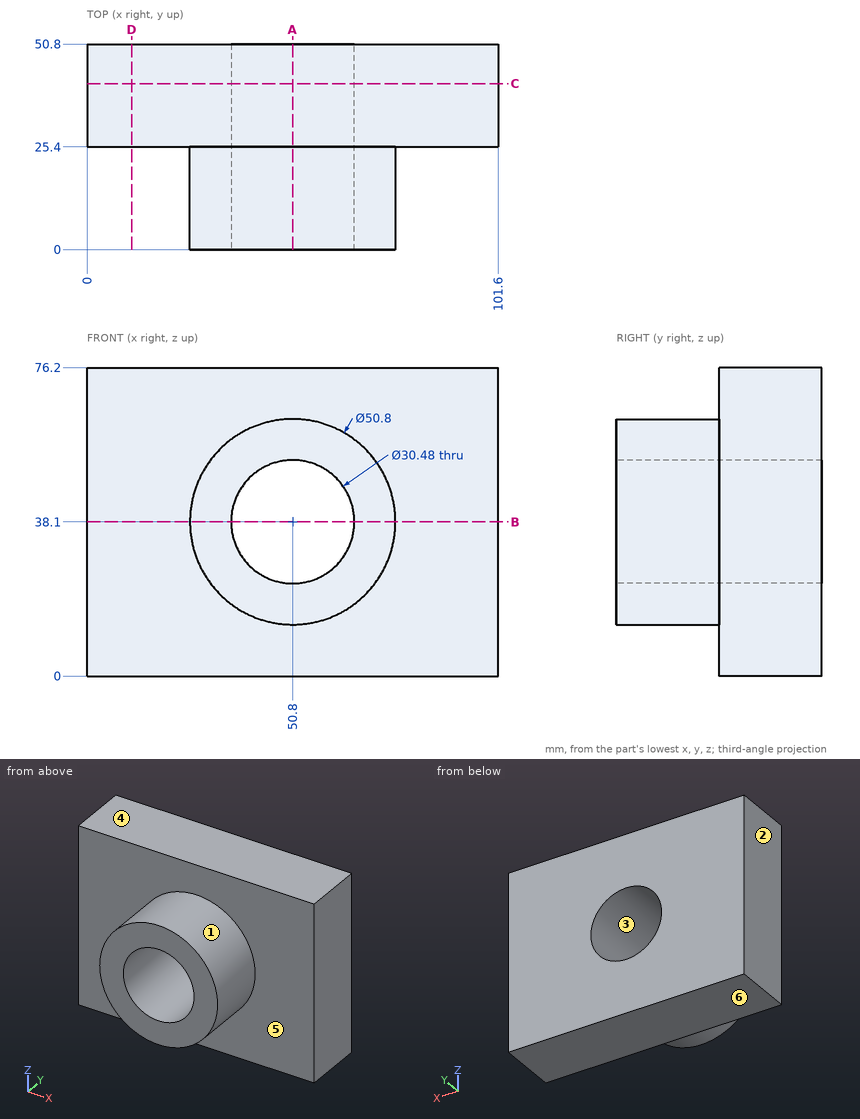
Print and shaded views of the part. All mm, measured from the part's lowest x, y and z. A direction names the side the tool comes from. Round coordinates to 2 decimals unless told otherwise and drop trailing zeros. Order: outer loops, then holes, each group sorted by start corner. A loop starts at its lowest first (then second) coordinate and runs counter-clockwise, first axis right, second up.
Q1. Slice it at D-D (x = 11). Write the cut outline in (y, z).
Q2. Slice it at C-C (y = 41). Write the cut outline in (x, z).
Q3. Drop flat-ended pins along their axis: pin 1 (4 mm diameter, centred on y = 18, z = 53, fed in from +X); pin 2 (24.5 mm diameter, centred on x = 50.8, z = 38.1, fed in from -Y); pin 3 (1.5 mm diameter, centred on y = 23, z = 54.5, fed in from -X). Give the stop position or say it passes through.
Q4. Wall check: L1, parallel to Z at x = 50.8, y = 35.5; L2, parallel to X at y = 19, z = 38; L3, parallel to Y at x = 25, z = 26.5. Give the ranges that are in metal, low to high.
Q5. Slice it at A-A (x = 50.8). Write the cut outline in (y, z), and give its area (3 significant figures).
Q6. Two-plate mould, pull along X, no slides. Class the marked faces 1, 2, 3 and 4: pulls with the +X half, pulls with the -X half, needs draft (parallel to the pull), parting line crosses it, or undercut.
Q7. Slice it at B-B (z = 38.1). Write the cut outline in (x, y), and give its area (3 significant figures).
Q8. Which spindle directions (+Z, -Z, +X, -X, +Y, -Y) get a long thin tool onto all of the face, cutting with end or side? Do the marked faces 5 and 6. Say none if no direction does.
Results below:
1. outline: (25.4, 0) - (50.8, 0) - (50.8, 76.2) - (25.4, 76.2) - close
2. outline: (0, 0) - (101.6, 0) - (101.6, 76.2) - (0, 76.2) - close; hole circle Ø30.48 at (50.8, 38.1)
3. pin 1: stops at x = 72.68
3. pin 2: passes through
3. pin 3: stops at x = 30.79
4. L1: z = 0 to 22.86, 53.34 to 76.2
4. L2: x = 25.4 to 35.56, 66.04 to 76.2
4. L3: y = 25.4 to 50.8
5. outline: (0, 12.7) - (25.4, 12.7) - (25.4, 0) - (50.8, 0) - (50.8, 22.86) - (0, 22.86) - close; (0, 53.34) - (50.8, 53.34) - (50.8, 76.2) - (25.4, 76.2) - (25.4, 63.5) - (0, 63.5) - close
5. area: 1,680 mm2
6. face 1: parting line crosses it
6. face 2: pulls with the -X half
6. face 3: undercut
6. face 4: needs draft
7. outline: (0, 25.4) - (25.4, 25.4) - (25.4, 0) - (35.56, 0) - (35.56, 50.8) - (0, 50.8) - close; (66.04, 0) - (76.2, 0) - (76.2, 25.4) - (101.6, 25.4) - (101.6, 50.8) - (66.04, 50.8) - close
7. area: 2,320 mm2
8. face 5: -Y
8. face 6: -Z, +X, -X, +Y, -Y
